from build123d import *

# Parameters (mm, degrees)
PAD_DEPTH       = 12.5
PAD001_DEPTH    = 10
PAD002_DEPTH    = 20
CHAMFER_SIZE    = 1
CHAMFER001_SIZE = 1
CHAMFER002_SIZE = 3.5


with BuildPart() as part:
    # Sketch → Pad (new body)
    with BuildSketch(Plane.XY):
        Polygon((0, 0), (16, 0), (16, -36), (12, -36), (0, -8), align=None)
    extrude(amount=PAD_DEPTH)

    # Sketch001 (on Face1 of Pad) → Pad001 (join)
    with BuildSketch(Plane(origin=(0, 0, 0), x_dir=(-1, 0, 0), z_dir=(0, 1, 0))):
        Polygon((-5.411165, 0), (-1.75, 3.661165), (-1.75, 8.838835), (-5.411165, 12.5), (-10.588835, 12.5), (-14.25, 8.838835), (-14.25, 3.661165), (-10.588835, 0), align=None)
    extrude(amount=PAD001_DEPTH)

    # Sketch002 (on Face12 of Pad001) → Pad002 (join)
    with BuildSketch(Plane.YZ.offset(16)):
        Polygon((-25.411165, 0), (-21.75, 3.661165), (-21.75, 8.838835), (-25.411165, 12.5), (-30.588835, 12.5), (-34.25, 8.838835), (-34.25, 3.661165), (-30.588835, 0), align=None)
    extrude(amount=PAD002_DEPTH)

    # Chamfer
    chamfer_edges = [part.edges().sort_by_distance(p)[0] for p in [
        (3.580583, 10, 1.830583),
        (1.75, 10, 6.25),
        (3.580583, 10, 10.669417),
        (8, 10, 12.5),
        (12.419417, 10, 10.669417),
        (14.25, 10, 6.25),
        (12.419417, 10, 1.830583),
        (8, 10, 0),
    ]]
    chamfer(chamfer_edges, length=CHAMFER_SIZE)

    # Chamfer001
    chamfer001_edges = [part.edges().sort_by_distance(p)[0] for p in [
        (36, -23.580583, 1.830583),
        (36, -21.75, 6.25),
        (36, -23.580583, 10.669417),
        (36, -28, 12.5),
        (36, -32.419417, 10.669417),
        (36, -34.25, 6.25),
        (36, -32.419417, 1.830583),
        (36, -28, 0),
    ]]
    chamfer(chamfer001_edges, length=CHAMFER001_SIZE)

    # Chamfer002
    chamfer002_edges = [part.edges().sort_by_distance(p)[0] for p in [
        (6, -22, 0),
        (6, -22, 12.5),
    ]]
    chamfer(chamfer002_edges, length=CHAMFER002_SIZE)


solid = part.part
Geometry: final body of the model. Coordinates: model frame, mm. A direction names the side the tool comes from. Coordinates: 2 decimals unless noted, no trailing zeros. Loops run counter-clockwise (first coordinate to the right, second up) from the corner with the lowest first, then second, coordinate; pieces in that order, holes last. Notation, with made-up numbers: M -30.5,-14.75 L -7.5,-14.75 A16 ccw -7.5,-9.75 Z; hole C 63.5,45 d9. An arc over 180 degrees is marked long. One line per item, written item: value. Start each with the question number.
1) Reachability of faces 1 (the flat face through (3.61, 4.44, 1.8)), 2 (the flat face through (25, -21.75, 6)), 3 (the flat face through (12.45, 4.44, 1.86)) from +Z, -Z, +X, -X, +Y, -Y: full face, straight path, thin tool, end or side. Return the list, or none.
2) Cut plane A-A (z = 6). Return loops of the section in (x, y).
3) Material intervals for L1, parallel to Y at x = 14.5, z = 4.5; L2, parallel to X at y = 2, z = 8; L3, parallel to Y at x = 31.5, z = 5.5, sorted ascending. Write a range as from..to.
4) Pin query (flat end, axial travel): P1, Ø4, axis at x = 21, z = 6, coming from the -Y side; P2, Ø6, axis at x = 8.5, z = 8.5, coming from the -Y side; P3, Ø4, axis at x = 29, z = 6, coming from the +Y side. Return the tip coordinate at first contact, or that it passes through.
5) Cut plane C-C (y = 5). Return loops of the section in (x, z).
6) Cut plane B-B (x = 31.5). Return loops of the section in (y, z), then the cut area to 3 significant figures.
7) Cut plane D-D (z = 2.75). Return loops of the section in (x, y).
Evaluation:
1. face 1: -Z, -X, +Y
1. face 2: +Z, -Z, +X, +Y
1. face 3: -Z, +X, +Y
2. outline: M 0,-8 L 12,-36 L 16,-36 L 16,-34.25 L 35,-34.25 L 36,-33.25 L 36,-22.75 L 35,-21.75 L 16,-21.75 L 16,0 L 14.25,0 L 14.25,9 L 13.25,10 L 2.75,10 L 1.75,9 L 1.75,0 L 0,0 Z
3. L1: -36..0
3. L2: 1.75..14.25
3. L3: -34.25..-21.75
4. P1: y = -34.25
4. P2: y = -34.83
4. P3: y = -21.75
5. outline: M 1.75,3.66 L 5.41,0 L 10.59,0 L 14.25,3.66 L 14.25,8.84 L 10.59,12.5 L 5.41,12.5 L 1.75,8.84 Z
6. outline: M -34.25,3.66 L -30.59,0 L -25.41,0 L -21.75,3.66 L -21.75,8.84 L -25.41,12.5 L -30.59,12.5 L -34.25,8.84 Z
6. area: 129 mm^2
7. outline: M 0,-6.1 L 12.82,-36 L 16,-36 L 16,-33.34 L 35,-33.34 L 36,-31.92 L 36,-24.08 L 35,-22.66 L 16,-22.66 L 16,0 L 13.34,0 L 13.34,9 L 11.92,10 L 4.08,10 L 2.66,9 L 2.66,0 L 0,0 Z
